Part model, mm, in its own coordinate system. Round coordinates to 2 decimals unless told otherwise and drop trailing zeros. Loops run counter-clockwise (first coordinate to the right, second up) from the corner with the lowest first, then second, coordinate; pieces in that order, holes last.
from build123d import *

# Parameters (mm, degrees)
F1_DEPTH = 12.5
F2_R     = 10
F3_DEPTH = 25
F5_DEPTH = 25


with BuildPart() as f1:
    # F0 (on Front) → F1 (new body, symmetric)
    with BuildSketch(Plane.XZ):
        Polygon((-54.605159, -18.751266), (-11.063506, -56.665088), (43.541652, -37.913821), (54.605159, 18.751266), (11.063506, 56.665088), (-43.541652, 37.913821), align=None)
    extrude(amount=F1_DEPTH, both=True)

    # F2 (on face) → F3 (cut)
    with BuildSketch(Plane.XZ.offset(12.5)):
        with Locations((5.531753, 28.332544)):
            Circle(F2_R)
        with Locations((27.302579, 9.375633)):
            Circle(F2_R)
        with Locations((21.770826, -18.956911)):
            Circle(F2_R)
        with Locations((-5.531753, -28.332544)):
            Circle(F2_R)
        with Locations((-27.302579, -9.375633)):
            Circle(F2_R)
        with Locations((-21.770826, 18.956911)):
            Circle(F2_R)
    extrude(amount=-F3_DEPTH, mode=Mode.SUBTRACT)

    # F4 (on face) → F5 (cut)
    with BuildSketch(Plane.XZ.offset(12.5)):
        with BuildLine():
            ThreePointArc((2.487469, 12.25), (0, 10), (-2.487469, 12.25))
            ThreePointArc((-2.487469, 12.25), (-2.598896, 12.226845), (-2.710108, 12.202676))
            ThreePointArc((-2.710108, 12.202676), (-4.067366, 9.135455), (-7.254939, 10.179187))
            ThreePointArc((-7.254939, 10.179187), (-7.347316, 10.112712), (-7.439083, 10.045399))
            ThreePointArc((-7.439083, 10.045399), (-7.431448, 6.691306), (-10.767965, 6.348301))
            ThreePointArc((-10.767965, 6.348301), (-10.825318, 6.25), (-10.881772, 6.151181))
            ThreePointArc((-10.881772, 6.151181), (-9.510565, 3.09017), (-12.419112, 1.419735))
            ThreePointArc((-12.419112, 1.419735), (-12.431524, 1.306606), (-12.442904, 1.193368))
            ThreePointArc((-12.442904, 1.193368), (-9.945219, -1.045285), (-11.922882, -3.754316))
            ThreePointArc((-11.922882, -3.754316), (-11.888206, -3.862712), (-11.852546, -3.970789))
            ThreePointArc((-11.852546, -3.970789), (-8.660254, -5), (-9.365077, -8.279211))
            ThreePointArc((-9.365077, -8.279211), (-9.28931, -8.364133), (-9.212774, -8.448361))
            ThreePointArc((-9.212774, -8.448361), (-5.877853, -8.09017), (-5.187965, -11.372556))
            ThreePointArc((-5.187965, -11.372556), (-5.084208, -11.419318), (-4.98003, -11.465134))
            ThreePointArc((-4.98003, -11.465134), (-2.079117, -9.781476), (-0.113807, -12.499482))
            ThreePointArc((-0.113807, -12.499482), (0, -12.5), (0.113807, -12.499482))
            ThreePointArc((0.113807, -12.499482), (2.079117, -9.781476), (4.98003, -11.465134))
            ThreePointArc((4.98003, -11.465134), (5.084208, -11.419318), (5.187965, -11.372556))
            ThreePointArc((5.187965, -11.372556), (5.877853, -8.09017), (9.212774, -8.448361))
            ThreePointArc((9.212774, -8.448361), (9.28931, -8.364133), (9.365077, -8.279211))
            ThreePointArc((9.365077, -8.279211), (8.660254, -5), (11.852545, -3.970789))
            ThreePointArc((11.852545, -3.970789), (11.888206, -3.862712), (11.922882, -3.754316))
            ThreePointArc((11.922882, -3.754316), (9.945219, -1.045285), (12.442904, 1.193368))
            ThreePointArc((12.442904, 1.193368), (12.431524, 1.306606), (12.419112, 1.419735))
            ThreePointArc((12.419112, 1.419735), (9.510565, 3.09017), (10.881772, 6.151181))
            ThreePointArc((10.881772, 6.151181), (10.825318, 6.25), (10.767965, 6.348301))
            ThreePointArc((10.767965, 6.348301), (7.431448, 6.691306), (7.439083, 10.045399))
            ThreePointArc((7.439083, 10.045399), (7.347316, 10.112712), (7.25494, 10.179187))
            ThreePointArc((7.25494, 10.179187), (4.067366, 9.135455), (2.710108, 12.202676))
            ThreePointArc((2.710108, 12.202676), (2.598896, 12.226845), (2.487469, 12.25))
        make_face()
    extrude(amount=-F5_DEPTH, mode=Mode.SUBTRACT)


solid = f1.part
1) Drop flat-ended pins along their axis: pin 1 Ø6 at (x, y) = (13, 3.5) entering from -Z; pin 2 Ø6 at (x, y) = (-32, -8) entering from -Z; pin 3 Ø10 at (y, z) = (-5, -23) entering from -X. Give the stop position or say it passes through.
Values:
pin 1: stops at z = -49.43
pin 2: stops at z = -41.05
pin 3: stops at x = -54.61
2) Slice it at C-C, the plane x = 47.5. Give the cut face in (y, z), then the cut area to 3 significant figures.
Values:
outline: (-12.5, -17.64) - (12.5, -17.64) - (12.5, 24.94) - (-12.5, 24.94) - close
area: 1,060 mm2
3) Slice it at D-D, the plane y = -0.75. Give the number of separate pieces and of enclosed holes in the cut face, then the cut area to 3 significant figures.
Values:
separate pieces: 1
enclosed holes: 7
area: 6,430 mm2
4) Slice it at A-A, the plane z = -26. Give the cut face in (x, y), then the cut area to 3 significant figures.
Values:
outline: (-46.28, -12.5) - (-15.26, -12.5) - (-15.26, 12.5) - (-46.28, 12.5) - close; (4.19, -12.5) - (14.67, -12.5) - (14.67, 12.5) - (4.19, 12.5) - close; (28.87, -12.5) - (45.87, -12.5) - (45.87, 12.5) - (28.87, 12.5) - close
area: 1,460 mm2
5) Slice it at B-B, the plane x = -30. Give the cut face in (y, z).
Values:
outline: (-12.5, -40.18) - (12.5, -40.18) - (12.5, -19) - (-12.5, -19) - close; (-12.5, 0.25) - (12.5, 0.25) - (12.5, 13.28) - (-12.5, 13.28) - close; (-12.5, 24.64) - (12.5, 24.64) - (12.5, 42.56) - (-12.5, 42.56) - close
6) Wall check: line 1 along Z through (x, y) = (-20, -2); line 2 along Z through (x, y) = (-21, 2); line 3 along X through (y, z) = (-6, 25.5). Give the ranges that are in metal, low to high.
Values:
line 1: z = -48.88 to -16.21, -2.54 to 9.11, 28.8 to 46
line 2: z = -48.01 to -17.14, -1.61 to 8.99, 28.93 to 45.65
line 3: x = -45.97 to -29.33, -14.21 to -4.06, 15.12 to 46.85
